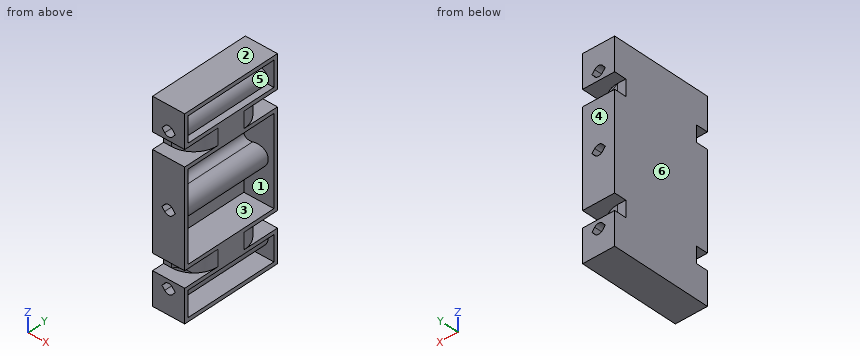
```python
from build123d import *

# Parameters (mm, degrees)
SKETCH1_W                    = 76.2
SKETCH1_H                    = 39.878
BOSS_EXTRUDE1_DEPTH          = 12.7
SKETCH2_W                    = 6.35
SKETCH2_H                    = 4.7625
CUT_EXTRUDE1_DEPTH           = 45.83819489
F_10_32_TAPPED_HOLE1_D       = 4.0386
FILLET1_R                    = 9.525
SKETCH6_W                    = 34.544
SKETCH6_H                    = 36.83
CUT_EXTRUDE3_DEPTH           = 9.525
CUT_EXTRUDE3_DRAFT           = -15
SKETCH6_W_2                  = 9.906
CUT_EXTRUDE3_PROFILE_2_DEPTH = 9.525
CUT_EXTRUDE3_PROFILE_2_DRAFT = -15
CUT_EXTRUDE3_PROFILE_3_DEPTH = 9.525
CUT_EXTRUDE3_PROFILE_3_DRAFT = -15
SKETCH7_R                    = 4.5593
SKETCH7_R_2                  = 2.0193
EXTRUDE_THIN1_DEPTH          = 39.878
DELETEFACE1_START            = 18.796
DELETEFACE1_DEPTH            = 6.35
DELETEFACE1_START_2          = -25.146
DELETEFACE1_2_DEPTH          = 6.35
FILLET2_R                    = 2.54
CUT_EXTRUDE4_DEPTH           = 57.596421146


with BuildPart() as part:
    # Sketch1 → Boss-Extrude1 (new body)
    with BuildSketch(Plane(origin=(0, 0, 0), x_dir=(0, 0, -1), z_dir=(1, 0, 0))):
        Rectangle(SKETCH1_W, SKETCH1_H)
    extrude(amount=BOSS_EXTRUDE1_DEPTH)

    # Sketch2 → Cut-Extrude1 (cut, through all)
    with BuildSketch(Plane(origin=(12.7, 0, 0), x_dir=(0, 0, -1), z_dir=(1, 0, 0))):
        with Locations((-21.971, 17.55775)):
            Rectangle(SKETCH2_W, SKETCH2_H)
        with Locations((21.971, 17.55775)):
            Rectangle(SKETCH2_W, SKETCH2_H)
        with Locations((-21.971, -17.55775)):
            Rectangle(SKETCH2_W, SKETCH2_H)
        with Locations((21.971, -17.55775)):
            Rectangle(SKETCH2_W, SKETCH2_H)
    extrude(amount=-CUT_EXTRUDE1_DEPTH, mode=Mode.SUBTRACT)

    # #10-32 Tapped Hole1 (through all)
    with Locations(Plane(origin=(0, 19.939, 0), x_dir=(1, 0, 0), z_dir=(0, 1, 0))):
        with Locations((6.35, 28.575), (6.35, 0), (6.35, -28.575)):
            Hole(F_10_32_TAPPED_HOLE1_D / 2)

    # Fillet1
    fillet1_edges = [part.edges().sort_by_distance(p)[0] for p in [
        (12.7, 15.1765, -21.971),
        (12.7, -15.1765, 21.971),
        (12.7, -15.1765, -21.971),
        (12.7, 15.1765, 21.971),
    ]]
    fillet(fillet1_edges, radius=FILLET1_R)


with BuildPart() as cut_extrude3_tool:
    # Sketch6 → Cut-Extrude3 (with draft: the straight prism first)
    with BuildSketch(Plane(origin=(12.7, 0, 0), x_dir=(0, 0, -1), z_dir=(1, 0, 0))):
        Rectangle(SKETCH6_W, SKETCH6_H)
    extrude(amount=-CUT_EXTRUDE3_DEPTH)
    # Cut-Extrude3: the draft: its side faces are tilted about the plane it starts from
    cut_extrude3_sides = [cut_extrude3_tool.faces().sort_by_distance(p)[0] for p in [
        (7.9375, 0, 17.272),
        (7.9375, -18.415, 0),
        (7.9375, 0, -17.272),
        (7.9375, 18.415, 0),
    ]]
    draft(cut_extrude3_sides, Plane(origin=(12.7, 0, 0), x_dir=(0, 0, -1), z_dir=(1, 0, 0)), CUT_EXTRUDE3_DRAFT)


with BuildPart() as part_1:
    add(part.part)

    # Cut-Extrude3: cut by cut_extrude3_tool
    add(cut_extrude3_tool.part, mode=Mode.SUBTRACT)


with BuildPart() as cut_extrude3_profile_2_tool:
    # Sketch6 → Cut-Extrude3 profile 2 (with draft: the straight prism first)
    with BuildSketch(Plane(origin=(12.7, 0, 0), x_dir=(0, 0, -1), z_dir=(1, 0, 0))):
        with Locations((31.623, 0)):
            Rectangle(SKETCH6_W_2, SKETCH6_H)
    extrude(amount=-CUT_EXTRUDE3_PROFILE_2_DEPTH)
    # Cut-Extrude3 profile 2: the draft: its side faces are tilted about the plane it starts from
    cut_extrude3_profile_2_sides = [cut_extrude3_profile_2_tool.faces().sort_by_distance(p)[0] for p in [
        (7.9375, 0, -26.67),
        (7.9375, -18.415, -31.623),
        (7.9375, 0, -36.576),
        (7.9375, 18.415, -31.623),
    ]]
    draft(cut_extrude3_profile_2_sides, Plane(origin=(12.7, 0, 0), x_dir=(0, 0, -1), z_dir=(1, 0, 0)), CUT_EXTRUDE3_PROFILE_2_DRAFT)


with BuildPart() as part_2:
    add(part_1.part)

    # Cut-Extrude3 profile 2: cut by cut_extrude3_profile_2_tool
    add(cut_extrude3_profile_2_tool.part, mode=Mode.SUBTRACT)


with BuildPart() as cut_extrude3_profile_3_tool:
    # Sketch6 → Cut-Extrude3 profile 3 (with draft: the straight prism first)
    with BuildSketch(Plane(origin=(12.7, 0, 0), x_dir=(0, 0, -1), z_dir=(1, 0, 0))):
        with Locations((-31.623, 0)):
            Rectangle(SKETCH6_W_2, SKETCH6_H)
    extrude(amount=-CUT_EXTRUDE3_PROFILE_3_DEPTH)
    # Cut-Extrude3 profile 3: the draft: its side faces are tilted about the plane it starts from
    cut_extrude3_profile_3_sides = [cut_extrude3_profile_3_tool.faces().sort_by_distance(p)[0] for p in [
        (7.9375, 0, 36.576),
        (7.9375, -18.415, 31.623),
        (7.9375, 0, 26.67),
        (7.9375, 18.415, 31.623),
    ]]
    draft(cut_extrude3_profile_3_sides, Plane(origin=(12.7, 0, 0), x_dir=(0, 0, -1), z_dir=(1, 0, 0)), CUT_EXTRUDE3_PROFILE_3_DRAFT)


with BuildPart() as part_3:
    add(part_2.part)

    # Cut-Extrude3 profile 3: cut by cut_extrude3_profile_3_tool
    add(cut_extrude3_profile_3_tool.part, mode=Mode.SUBTRACT)

    # Sketch7 → Extrude-Thin1 (add, through all)
    # profile 1 of 3: a face of its own
    with BuildSketch(Plane(origin=(0, 19.939, 0), x_dir=(1, 0, 0), z_dir=(0, 1, 0))):
        with Locations((6.35, -28.575)):
            Circle(SKETCH7_R)
        with Locations((6.35, -28.575)):
            Circle(SKETCH7_R_2, mode=Mode.SUBTRACT)
    # profile 2 of 3: a face of its own
    with BuildSketch(Plane(origin=(0, 19.939, 0), x_dir=(1, 0, 0), z_dir=(0, 1, 0))):
        with Locations((6.35, 0)):
            Circle(SKETCH7_R)
        with Locations((6.35, 0)):
            Circle(SKETCH7_R_2, mode=Mode.SUBTRACT)
    # profile 3 of 3: a face of its own
    with BuildSketch(Plane(origin=(0, 19.939, 0), x_dir=(1, 0, 0), z_dir=(0, 1, 0))):
        with Locations((6.35, 28.575)):
            Circle(SKETCH7_R)
        with Locations((6.35, 28.575)):
            Circle(SKETCH7_R_2, mode=Mode.SUBTRACT)
    extrude(amount=-EXTRUDE_THIN1_DEPTH)

    # DeleteFace1: read off the stored shape, not the designer's step
    # DeleteFace1 outline → DeleteFace1 (cut)
    with BuildSketch(Plane.XY.offset(DELETEFACE1_START)):
        with BuildLine():
            ThreePointArc((3.175, 15.1765), (9.910192091, 12.386692091), (12.7, 5.6515))
            Line((12.7, 5.6515), (12.7, 19.939))
            Line((12.7, 19.939), (0, 19.939))
            Line((0, 19.939), (0, 15.1765))
            Line((0, 15.1765), (3.175, 15.1765))
        make_face()
        with BuildLine():
            Line((12.7, -19.939), (12.7, -5.6515))
            ThreePointArc((12.7, -5.6515), (9.910192091, -12.386692091), (3.175, -15.1765))
            Line((3.175, -15.1765), (0, -15.1765))
            Line((0, -15.1765), (0, -19.939))
            Line((0, -19.939), (12.7, -19.939))
        make_face()
    extrude(amount=DELETEFACE1_DEPTH, mode=Mode.SUBTRACT)

    # DeleteFace1 2 outline → DeleteFace1 2 (cut)
    with BuildSketch(Plane.XY.offset(DELETEFACE1_START_2)):
        with BuildLine():
            ThreePointArc((3.175, 15.1765), (9.910192091, 12.386692091), (12.7, 5.6515))
            Line((12.7, 5.6515), (12.7, 19.939))
            Line((12.7, 19.939), (0, 19.939))
            Line((0, 19.939), (0, 15.1765))
            Line((0, 15.1765), (3.175, 15.1765))
        make_face()
        with BuildLine():
            Line((12.7, -19.939), (12.7, -5.6515))
            ThreePointArc((12.7, -5.6515), (9.910192091, -12.386692091), (3.175, -15.1765))
            Line((3.175, -15.1765), (0, -15.1765))
            Line((0, -15.1765), (0, -19.939))
            Line((0, -19.939), (12.7, -19.939))
        make_face()
    extrude(amount=DELETEFACE1_2_DEPTH, mode=Mode.SUBTRACT)

    # Fillet2
    # the kernel refuses this fillet: 2.54 mm, written as the material it adds along each edge
    with BuildSketch(Plane(origin=(3.175, -25.359661976, -3.27209283), x_dir=(0, 0, -1), z_dir=(0, 1, 0))) as fillet2_piece_1_section:
        with BuildLine():
            CenterArc((3.798751213, -2.54), FILLET2_R, 90, 95.131704374)
            ThreePointArc((1.268932235, -2.767191413), (0.872245463, -1.274558842), (0, 0))
            Line((0, 0), (3.798751213, 0))
        make_face()
    fillet2_piece_1 = extrude(amount=50.719323951, mode=Mode.PRIVATE)
    fillet2_piece_1 = split(fillet2_piece_1, bisect_by=Plane(origin=(5.549219508, -16.498954142, -3.27209283), z_dir=(0.25881904510252135, 0.9659258262890681, 0)), keep=Keep.TOP, mode=Mode.PRIVATE)
    fillet2_piece_1 = split(fillet2_piece_1, bisect_by=Plane(origin=(-7.130611479, 13.101403669, -3.27209283), z_dir=(0.25881904510252135, -0.9659258262890681, 0)), keep=Keep.TOP, mode=Mode.PRIVATE)
    add(fillet2_piece_1)
    with BuildSketch(Plane(origin=(3.175, -25.359661976, 3.27209283), x_dir=(0.9089856543258207, 0, 0.4168273986074566), z_dir=(0, 1, 0))) as fillet2_piece_2_section:
        with BuildLine():
            CenterArc((3.892247148, -2.394268765), FILLET2_R, 109.502744929, 95.131704374)
            Line((1.583423586, -3.453010357), (0, 0))
            ThreePointArc((0, 0), (1.52213151, -0.261587567), (3.04426302, 0))
        make_face()
    fillet2_piece_2 = extrude(amount=50.719323951, mode=Mode.PRIVATE)
    fillet2_piece_2 = split(fillet2_piece_2, bisect_by=Plane(origin=(5.549219508, -16.498954142, 3.27209283), z_dir=(0.25881904510252135, 0.9659258262890681, 0)), keep=Keep.TOP, mode=Mode.PRIVATE)
    fillet2_piece_2 = split(fillet2_piece_2, bisect_by=Plane(origin=(-7.130611479, 13.101403669, 3.27209283), z_dir=(0.25881904510252135, -0.9659258262890681, 0)), keep=Keep.TOP, mode=Mode.PRIVATE)
    add(fillet2_piece_2)
    with BuildSketch(Plane(origin=(3.175, -22.657937307, -31.84709283), x_dir=(0, 0, -1), z_dir=(0, 1, 0))) as fillet2_piece_3_section:
        with BuildLine():
            CenterArc((3.73080949, -2.009058502), FILLET2_R, 127.723943203, 61.728755264)
            ThreePointArc((1.225298821, -2.426211095), (0.797654993, -1.119672984), (0, 0))
            Line((0, 0), (2.176691112, 0))
        make_face()
    fillet2_piece_3 = extrude(amount=45.315874614, mode=Mode.PRIVATE)
    fillet2_piece_3 = split(fillet2_piece_3, bisect_by=Plane(origin=(4.873788341, -16.317972906, -31.84709283), z_dir=(0.25881904510252135, 0.9659258262890681, 0)), keep=Keep.TOP, mode=Mode.PRIVATE)
    fillet2_piece_3 = split(fillet2_piece_3, bisect_by=Plane(origin=(-6.455180312, 13.282384904, -31.84709283), z_dir=(0.25881904510252135, -0.9659258262890681, 0)), keep=Keep.TOP, mode=Mode.PRIVATE)
    add(fillet2_piece_3)
    with BuildSketch(Plane(origin=(3.175, -22.657937307, 31.84709283), x_dir=(0.8926255836617852, 0, 0.4507988103272426), z_dir=(0, 1, 0))) as fillet2_piece_4_section:
        with BuildLine():
            CenterArc((3.475181498, -2.424534816), FILLET2_R, 107.342247882, 61.728755264)
            Line((0.981249764, -1.942970174), (0, 0))
            ThreePointArc((0, 0), (1.359030673, -0.207260005), (2.718061346, 0))
        make_face()
    fillet2_piece_4 = extrude(amount=45.315874614, mode=Mode.PRIVATE)
    fillet2_piece_4 = split(fillet2_piece_4, bisect_by=Plane(origin=(-6.455180312, 13.282384904, 31.84709283), z_dir=(0.25881904510252135, -0.9659258262890681, 0)), keep=Keep.TOP, mode=Mode.PRIVATE)
    fillet2_piece_4 = split(fillet2_piece_4, bisect_by=Plane(origin=(4.873788341, -16.317972906, 31.84709283), z_dir=(0.25881904510252135, 0.9659258262890681, 0)), keep=Keep.TOP, mode=Mode.PRIVATE)
    add(fillet2_piece_4)

    # Sketch8 → Cut-Extrude4 (cut, through all)
    with BuildSketch(Plane.XZ.offset(19.939)):
        with BuildLine():
            Line((8.986008939, 28.575), (7.896873544, 29.87298102))
            ThreePointArc((7.896873544, 29.87298102), (6.35, 30.5943), (4.803126456, 29.87298102))
            Line((4.803126456, 29.87298102), (3.713991061, 28.575))
            Line((3.713991061, 28.575), (4.803126456, 27.27701898))
            ThreePointArc((4.803126456, 27.27701898), (6.35, 26.5557), (7.896873544, 27.27701898))
            Line((7.896873544, 27.27701898), (8.986008939, 28.575))
        make_face()
        with BuildLine():
            Line((8.986008939, 0), (7.896873544, 1.29798102))
            ThreePointArc((7.896873544, 1.29798102), (6.35, 2.0193), (4.803126456, 1.29798102))
            Line((4.803126456, 1.29798102), (3.713991061, 0))
            Line((3.713991061, 0), (4.803126456, -1.29798102))
            ThreePointArc((4.803126456, -1.29798102), (6.35, -2.0193), (7.896873544, -1.29798102))
            Line((7.896873544, -1.29798102), (8.986008939, 0))
        make_face()
        with BuildLine():
            Line((8.986008939, -28.575), (7.896873544, -27.27701898))
            ThreePointArc((7.896873544, -27.27701898), (6.35, -26.5557), (4.803126456, -27.27701898))
            Line((4.803126456, -27.27701898), (3.713991061, -28.575))
            Line((3.713991061, -28.575), (4.803126456, -29.87298102))
            ThreePointArc((4.803126456, -29.87298102), (6.35, -30.5943), (7.896873544, -29.87298102))
            Line((7.896873544, -29.87298102), (8.986008939, -28.575))
        make_face()
    extrude(amount=-CUT_EXTRUDE4_DEPTH, mode=Mode.SUBTRACT)


solid = part_3.part
```
The listing builds one solid part. Answer for the finished solid, in the listing's coordinates (mm). Face numbers are marked on the shaded views. A direction names the side the tool comes from. Round coordinates to 2 decimals unless told otherwise and drop trailing zeros. Loops run counter-clockwise (first coordinate to the right, second up) from the corner with the lowest first, then second, coordinate; pieces in that order, holes last. Notation, with made-up numbers: (75, 12.25) -> (85, 12.25) arc R13 cw to (85, 25.25) -> close; hole circle Ø2 at (-38.75, 87.5). An arc over 180 degrees is marked (long way). Use one line per item in the form item = value.
1. Flat-ended cylindrical pins translate along their axes: pin 1 Ø8.5 at (y, z) = (4.5, 9.5) entering from +X; pin 2 Ø3.5 at (x, z) = (2, 23) entering from -Y; pin 3 Ø3.5 at (x, z) = (2, -23) entering from +Y. Find the tip coordinate at first contact, or state that the pin passes through.
Answer key:
pin_1 = 3.94
pin_2 = -15.18
pin_3 = 15.18
2. A tool of negligible diameter and unlimited length cuts with its end or side. For the marked faces 1 and 2, from which of +Z, -Z, +X, -X, +Y, -Y can it reach the whole face along a straight path? Write none if from no direction.
Answer key:
face_1 = +X
face_2 = +Z, +X, -X, +Y, -Y
3. The part is cut by section B-B on y = 11. Give the number of separate pieces and of enclosed holes in the cut face, and give its area (3 significant figures).
Answer key:
separate_pieces = 1
enclosed_holes = 3
area = 593 mm²
4. For a pull along Y with two mould halves and no side action, classify the marked faces 3, 4, 5 and 6 as released by +Y, released by -Y, zero draft, split by the parting line, or undercut.
Answer key:
face_3 = undercut
face_4 = released by +Y
face_5 = undercut
face_6 = zero draft
5. The part is cut by section A-A on z = 32. Determine the outline of the cut face in (x, y) (3 decimals), and give its area (3 significant figures).
Answer key:
outline = (0, -19.939) -> (12.7, -19.939) -> (12.7, -18.415) -> (9.359, -17.52) -> (9.359, 17.52) -> (12.7, 18.415) -> (12.7, 19.939) -> (0, 19.939) -> close
area = 386 mm²
6. Find the intervals of material crossed by probe 1 along Z at (x, y) = (9.5, 11); probe 2 along Z at (x, y) = (11.25, 16); probe 3 along Z at (x, y) = (11, 4), in increasing order. Write a range as [from, to].
Answer key:
probe_1 = [-38.1, -35.72], [-31.87, -16.41], [-3.3, 3.3], [16.41, 31.87], [35.72, 38.1]
probe_2 = [-38.1, -36.19], [-27.06, -25.15], [-18.8, -16.88], [16.88, 18.8], [25.15, 27.06], [36.19, 38.1]
probe_3 = [-38.1, -36.12], [-27.13, -16.82], [16.82, 27.13], [36.12, 38.1]
